```python
from build123d import *

# Parameters (mm, degrees)
F1_DEPTH = 12.7
F2_W     = 25.4
F2_H     = 25.4
F3_DEPTH = 25.4
F4_R     = 5.08
F5_W     = 1.27
F5_H     = 5.08
F6_DEPTH = 15.24
F7_SIZE  = 1.524
F8_R     = 0.9525
F9_DEPTH = 127


with BuildPart() as f1:
    # F0 (on Top) → F1 (new body)
    with BuildSketch(Plane.XY):
        Polygon((-12.7, -25.4), (0, -25.4), (12.7, -25.4), (12.7, 0), (-12.7, 0), align=None)
        Polygon((6.368273, -21.585433), (0.018273, -21.585433), (-6.331727, -21.585433), (-6.331727, -17.140433), (6.368273, -17.140433), align=None, mode=Mode.SUBTRACT)
    extrude(amount=F1_DEPTH)

    # F2 (on face) → F3 (join)
    with BuildSketch(Plane.XY.offset(12.7)):
        with Locations((0, -12.7)):
            Rectangle(F2_W, F2_H)
    extrude(amount=F3_DEPTH)

    # F4
    f4_edges = [f1.edges().sort_by_distance(p)[0] for p in [
        (-12.7, -25.4, 19.05),
        (12.7, -25.4, 19.05),
        (-12.7, 0, 19.05),
        (12.7, 0, 19.05),
    ]]
    fillet(f4_edges, radius=F4_R)

    # F5 (on face) → F6 (join)
    with BuildSketch(Plane.XY.offset(38.1)):
        with Locations((-6.985, -11.095791)):
            Rectangle(F5_W, F5_H)
        with Locations((6.985, -11.095791)):
            Rectangle(F5_W, F5_H)
    extrude(amount=F6_DEPTH)

    # F7
    f7_edges = [f1.edges().sort_by_distance(p)[0] for p in [
        (-6.985, -13.635791, 53.34),
        (6.985, -13.635791, 53.34),
        (-6.985, -8.555791, 53.34),
        (6.985, -8.555791, 53.34),
    ]]
    chamfer(f7_edges, length=F7_SIZE)

    # F8 (on face) → F9 (cut)
    with BuildSketch(Plane(origin=(-7.62, 0, 0), x_dir=(0, -1, 0), z_dir=(-1, 0, 0))):
        with Locations((11.095791, 51.816)):
            Circle(F8_R)
    extrude(amount=-F9_DEPTH, mode=Mode.SUBTRACT)


solid = f1.part
```
Geometry: final body of the model. Coordinates: model frame, mm. A direction names the side the tool comes from. Round coordinates to 2 decimals unless told otherwise and drop trailing zeros. Order: outer loops, then holes, each group sorted by start corner. A loop starts at its lowest first (then second) coordinate and runs counter-clockwise, first axis right, second up. Notation, with made-up numbers: (86, 33.5) - (109, 33.5) arc R17 cw to (109, 43.5) - close; hole circle Ø2 at (-13.5, 45). An arc over 180 degrees is marked (long way). Write item = value, one per line. Start each with the question number.
Q1. Cut plane A-A on z = 42. Return the cut outline in (x, y), and give its area (3 significant figures).
Q2. Pin query (flat end, axial travel): pin 1 (1.3 mm diameter, centred on x = 0, y = -20.5, fed in from -Z); pin 2 (2.5 mm diameter, centred on y = -11, z = 43.5, fed in from +X); pin 3 (4 mm diameter, centred on y = -12.5, z = 44.5, fed in from -X); pin 4 (1.5 mm diameter, centred on y = -11.1, z = 51.82, fed in from -X). Return the tip coordinate at first contact, or that it passes through.
Q3. Cut plane B-B on x = -3. Return the cut outline in (y, z).
Q4. Cut plane D-D on y = -19. Return the cut outline in (x, z), and give its area (3 significant figures).
Q5. Pull-direction query (X, two-part tool) for faces 1 (the flat face through (-12.7, -13, 19)), 2 (the flat face through (6.368, -19, 6)), 3 (the flat face through (0, -13, 0)); classes: +X half, -X half, draft (parallel to the pull), parting line (faces both ways), or undercut.
Q6. Cut plane C-C on z = 8.5. Return the cut outline in (x, y), and give its area (3 significant figures).
Q7. Ray query, line 1 (X direction, y = -11, z = 50); line 2 (Y direction, x = -2.25, z = 6.5); line 3 (Z direction, x = -1.5, y = -17). Return the intervals inside material, ascending. Write a range as from..to.
Q8. Access query for faces 4 (the flat face through (-7, -8.556, 45)), 5 (the flat face through (0, -19, 12.7)), 6 (the flat face through (-7, -13.636, 45)). Directions: +Z, -Z, +X, -X, +Y, -Y. A direction counts if a zero-diameter tool reaches every point of the face in a straight line with its end or side. Return the directions, or none.
Outcome:
q1.outline = (-7.62, -13.64) - (-6.35, -13.64) - (-6.35, -8.56) - (-7.62, -8.56) - close; (6.35, -13.64) - (7.62, -13.64) - (7.62, -8.56) - (6.35, -8.56) - close
q1.area = 12.9 mm^2
q2.pin_1 = 12.7
q2.pin_2 = 7.62
q2.pin_3 = -7.62
q2.pin_4 = through
q3.outline = (-25.4, 0) - (-21.59, 0) - (-21.59, 12.7) - (-17.14, 12.7) - (-17.14, 0) - (0, 0) - (0, 38.1) - (-25.4, 38.1) - close
q4.outline = (-12.7, 0) - (-6.33, 0) - (-6.33, 12.7) - (6.37, 12.7) - (6.37, 0) - (12.7, 0) - (12.7, 38.1) - (-12.7, 38.1) - close
q4.area = 806 mm^2
q5.face_1 = -X half
q5.face_2 = undercut
q5.face_3 = draft
q6.outline = (-12.7, -20.32) arc R5.08 ccw to (-7.62, -25.4) - (7.62, -25.4) arc R5.08 ccw to (12.7, -20.32) - (12.7, -5.08) arc R5.08 ccw to (7.62, 0) - (-7.62, 0) arc R5.08 ccw to (-12.7, -5.08) - close; hole (-6.33, -21.59) - (6.37, -21.59) - (6.37, -17.14) - (-6.33, -17.14) - close
q6.area = 567 mm^2
q7.line_1 = -7.62..-6.35, 6.35..7.62
q7.line_2 = -25.4..-21.59, -17.14..0
q7.line_3 = 0..38.1
q8.face_4 = +Z, +X, -X, +Y
q8.face_5 = -Z
q8.face_6 = +Z, +X, -X, -Y
